Here's how the part is built. I have some questions about the finished solid (model axes, mm). A direction names the side the tool comes from. Round coordinates to 2 decimals unless told otherwise and drop trailing zeros. Write each loop counter-clockwise with the first axis right and the second up, starting at its lowest first coordinate (ties: lowest second). Pieces come first, ordered by that corner, then holes. Notation, with made-up numbers: (14.5, 77.5) - (65.5, 77.5) arc R12 cw to (65.5, 86.5) - close; hole circle Ø10 at (41, 54). An arc over 180 degrees is marked (long way). One line per item, written item: value. Start each with the question number.
Item 1: If I drill on line 1 (Z direction, x = -188, y = -308); line 2 (Y direction, x = -167.5, z = 572.5); line 3 (Z direction, x = -363.5, y = -509.5), over which ranges is the centre line in solid material (lowest first)?
Item 2: For faces 1 (the face through (-191, -610, 939.546)), 2 (the face through (-72, -610.13, 422.04)), 3 (the face through (-74.047, -37.567, 929.915)), 4 (the face through (-309, -37.57, 932.29)), 5 (the face through (-306.953, -610.133, 85.831)), which set-ups out of +Z, -Z, +X, -X, +Y, -Y let a thin tool reach every point of the face, with its end or its side?
Item 3: Thinking about a two-plate mould opening in Z: for faces 6 (the face through (-31, -76.2, 965)), 7 (the face through (-193, -647.7, 515)), 8 (the face through (-188, -610, 1015.746)), which applies, released by +Z, released by -Z, zero draft, split by the parting line, or undercut?
Item 4: Imagine slicing it at B-B, the plane z = 727. Please give me the cut outline in (x, y), then the cut area to 3 significant figures.
Item 5: Imagine slicing it at A-A, the plane y = -219.5. Count the separate pieces of the cut face and the enclosed holes in it, then the cut area to 3 significant figures.
Item 6: For P1, Ø5, axis at y = -272, z = 476.5, coming from the +X side; P2, Ø2, axis at x = -181.5, y = -104.5, coming from the -Z side; P3, Ø12, axis at x = -274.5, y = -285, coming from the -Z side, each with a flat end and sliding along its axis, tell me the tip position at first contact or that it passes through.
```python
from build123d import *

# Parameters (mm, degrees)
F1_DEPTH = 76.2
F2_R     = 31.75
F3_DEPTH = 247.65


# Not quite as in the source:
# - a feature names something its author has since deleted; it is built from what else it names


with BuildPart() as f1:
    # F0 (on Front) → F1 (new body)
    with BuildSketch(Plane.XZ):
        Polygon((-234.95, 507.873), (-190.5, 559.3963478261), (-292.1, 677.164), (-381, 677.164), align=None)
        Polygon((-190.5, 456.3496521739), (-146.05, 507.873), (-190.5, 559.3963478261), (-234.95, 507.873), align=None)
        Polygon((-190.5, 559.3963478261), (-146.05, 507.873), (0, 677.164), (-88.9, 677.164), align=None)
        Polygon((-88.9, 338.582), (0, 338.582), (-146.05, 507.873), (-190.5, 456.3496521739), align=None)
        Polygon((-381, 338.582), (-292.1, 338.582), (-190.5, 456.3496521739), (-234.95, 507.873), align=None)
        Polygon((-234.95, 169.291), (-190.5, 220.8143478261), (-292.1, 338.582), (-381, 338.582), align=None)
        Polygon((-190.5, 220.8143478261), (-146.05, 169.291), (0, 338.582), (-88.9, 338.582), align=None)
        Polygon((-190.5, 117.7676521739), (-146.05, 169.291), (-190.5, 220.8143478261), (-234.95, 169.291), align=None)
        Polygon((-88.9, 0), (0, 0), (-146.05, 169.291), (-190.5, 117.7676521739), align=None)
        Polygon((-292.1, 0), (-190.5, 117.7676521739), (-234.95, 169.291), (-381, 0), align=None)
        Polygon((-381, 677.164), (-292.1, 677.164), (-190.5, 794.9316521739), (-234.95, 846.455), align=None)
        Polygon((-190.5, 794.9316521739), (-146.05, 846.455), (-190.5, 897.9783478261), (-234.95, 846.455), align=None)
        Polygon((-88.9, 677.164), (0, 677.164), (-146.05, 846.455), (-190.5, 794.9316521739), align=None)
        Polygon((-190.5, 897.9783478261), (-146.05, 846.455), (0, 1015.746), (-88.9, 1015.746), (-154.6389347337, 939.546), align=None)
        Polygon((-154.6389347337, 939.546), (-88.9, 1015.746), (-292.1, 1015.746), (-226.3610652663, 939.546), align=None)
        Polygon((-234.95, 846.455), (-190.5, 897.9783478261), (-226.3610652663, 939.546), (-292.1, 1015.746), (-381, 1015.746), align=None)
    extrude(amount=F1_DEPTH)

    # F2 (on face) → F3 (join)
    with BuildSketch(Plane.XZ.offset(76.2)):
        with Locations((-336.55, 677.164)):
            Circle(F2_R)
        with Locations((-44.45, 677.164)):
            Circle(F2_R)
        with Locations((-190.5, 507.873)):
            Circle(F2_R)
        with Locations((-190.5, 169.291)):
            Circle(F2_R)
        with Locations((-44.45, 338.582)):
            Circle(F2_R)
        with Locations((-336.55, 338.582)):
            Circle(F2_R)
        with Locations((-190.5, 846.455)):
            Circle(F2_R)
        with Locations((-44.45, 977.646)):
            Circle(F2_R)
        with Locations((-139.7, 977.646)):
            Circle(F2_R)
        with Locations((-336.55, 977.646)):
            Circle(F2_R)
        with Locations((-241.3, 977.646)):
            Circle(F2_R)
    extrude(amount=F3_DEPTH)

    # F4: F1 across face


with BuildPart() as f1_1:
    add(f1.part)
    add(f1.part.mirror(Plane(origin=(-336.55, -323.85, 977.646), x_dir=(1, 0, 0), z_dir=(0, -1, 0))))


solid = f1_1.part
```
Values follow:
1. line 1: z = 137.64 to 200.94, 476.22 to 539.52, 814.8 to 878.11
1. line 2: y = -647.7 to -571.5, -76.2 to 0
1. line 3: z = 321.8 to 355.37, 660.38 to 693.95, 960.86 to 994.43
2. face 1: +Y, -Y
2. face 2: +X, +Y, -Y
2. face 3: +X, +Y
2. face 4: -X, +Y
2. face 5: -X, +Y, -Y
3. face 6: undercut
3. face 7: zero draft
3. face 8: released by +Z
4. outline: (-338.01, -647.7) - (-249.11, -647.7) - (-249.11, -571.5) - (-338.01, -571.5) - close; (-338.01, -76.2) - (-249.11, -76.2) - (-249.11, 0) - (-338.01, 0) - close; (-131.89, -647.7) - (-42.99, -647.7) - (-42.99, -571.5) - (-131.89, -571.5) - close; (-131.89, -76.2) - (-42.99, -76.2) - (-42.99, 0) - (-131.89, 0) - close
4. area: 27,100 mm^2
5. separate pieces: 11
5. enclosed holes: 0
5. area: 34,800 mm^2
6. P1: stops at x = -177.29
6. P2: stops at z = 138.57
6. P3: stops at z = 961.27
